For this review, take the finished solid that the model builds, in its own axes (mm). A direction names the side the tool comes from. Coordinates: 2 decimals unless noted, no trailing zeros. Loops run counter-clockwise (first coordinate to the right, second up) from the corner with the lowest first, then second, coordinate; pieces in that order, holes last. Notation, with made-up numbers: (-29, -11) - (-6, -11) arc R23 cw to (-6, -2) - close; hole circle Ø4 at (-2, -7). An arc over 180 degrees is marked (long way). Answer as a JSON object with one key per item and string values. Group by question number.
Item 1: Clearance check with flat-ended pins moving along their axes: pin 1 (24 mm diameter, centred on y = 115.5, z = 54, fed in from +X); pin 2 (24 mm diameter, centred on y = 120, z = 23, fed in from -X); pin 3 (2 mm diameter, centred on x = 43, y = 182, fed in from +Z). State where each tip first meets the part, or that it passes through.
Item 2: Tool access review of faces 1 (the flat face through (121.505, 144, 33)), 2 (the flat face through (120.005, 144, 33)), 3 (the flat face through (74, 147, 0)): name each direction out of +Z, -Z, +X, -X, +Y, -Y from which nothing blocks a thin tool from reaching the whole face with its end or side.
Item 3: To check wall thickness, follow line 1 (Z direction, x = 119, y = 234); line 2 (X direction, y = 171, z = 4.5). State the ranges of each line that lie inside material, in increasing order.
Item 4: We need section B-B (x = 103). Give the boundary of the cut face in (y, z), then the cut area to 3 significant figures.
Item 5: We need section A-A (y = 104.5). Give the boundary of the cut face in (x, z).
Item 6: We need section C-C (z = 45.5). Give the boundary of the cut face in (x, y), then the cut area to 3 significant figures.
from build123d import *

# Parameters (mm, degrees)
F0_W     = 150
F0_H     = 290
F1_DEPTH = 2
F2_W     = 1.5
F2_H     = 160
F3_DEPTH = 80
F5_DEPTH = 25


with BuildPart() as f1:
    # F0 (on Top) → F1 (new body)
    with BuildSketch(Plane.XY):
        with Locations((75, 145)):
            Rectangle(F0_W, F0_H)
    extrude(amount=F1_DEPTH)

    # F2 (on face) → F3 (join)
    with BuildSketch(Plane.XY.offset(2)):
        with Locations((120.755315, 145)):
            Rectangle(F2_W, F2_H)
    extrude(amount=F3_DEPTH)

    # F4 (on face) → F5 (cut)
    with BuildSketch(Plane.YZ.offset(121.505315)):
        with BuildLine():
            Line((65, 82), (65, 2))
            ThreePointArc((65, 2), (88.431458, 58.568542), (145, 82))
            Line((145, 82), (65, 82))
        make_face()
        with BuildLine():
            ThreePointArc((145, 82), (201.568542, 58.568542), (225, 2))
            Line((225, 2), (225, 82))
            Line((225, 82), (145, 82))
        make_face()
    extrude(amount=-F5_DEPTH, mode=Mode.SUBTRACT)


solid = f1.part
Check sheet entries:
{
 "1": {"pin 1": "stops at x = 121.51", "pin 2": "stops at x = 120.01", "pin 3": "stops at z = 2"},
 "2": {"face 1": "+Z, +X, +Y, -Y", "face 2": "+Z, -X, +Y, -Y", "face 3": "-Z, +X, -X, +Y, -Y"},
 "3": {"line 1": "z = 0 to 2", "line 2": "x = 120.01 to 121.51"},
 "4": {"outline": "(0, 0) - (290, 0) - (290, 2) - (0, 2) - close", "area": "580 mm2"},
 "5": {"outline": "(0, 0) - (150, 0) - (150, 2) - (121.51, 2) - (121.51, 70.99) - (120.01, 70.99) - (120.01, 2) - (0, 2) - close"},
 "6": {"outline": "(120.01, 77.86) - (121.51, 77.86) - (121.51, 212.14) - (120.01, 212.14) - close", "area": "201 mm2"}
}
